Geometry: final body of the model. Coordinates: model frame, mm. Face numbers are marked on the shaded views. A direction names the side the tool comes from. Give positions to 0.01 mm unless a question says otherwise; leave off trailing zeros. Write each loop counter-clockwise with the first axis right and the second up, starting at its lowest first coordinate (ties: lowest second). Pieces come first, ordered by that corner, then holes. Notation, with made-up numbers: (-17.5, 43) -> (11.5, 43) arc R22 cw to (11.5, 80) -> close; hole circle Ø7 at (46.25, -37.75). An arc over 180 degrees is marked (long way). Answer in a Markdown table with one row per item. Add a question column.
from build123d import *

# Parameters (mm, degrees)
BOSS_EXTRUDE1_DEPTH = 60
SKETCH6_W           = 76.2
SKETCH6_H           = 139.7
BOSS_EXTRUDE3_DEPTH = 3
SKETCH7_W           = 254.695348458
SKETCH7_H           = 135.329086622
CUT_EXTRUDE1_DEPTH  = 76.2
SKETCH8_W           = 10
SKETCH8_H           = 5
CUT_EXTRUDE2_DEPTH  = 95.039099262
SKETCH9_W           = 55
SKETCH9_H           = 40
CUT_EXTRUDE3_DEPTH  = 204.2
SKETCH10_W          = 200.764393162
SKETCH10_H          = 14.388440844
CUT_EXTRUDE4_DEPTH  = 15
BOSS_EXTRUDE4_DEPTH = 4
BOSS_EXTRUDE5_DEPTH = 4


with BuildPart() as part:
    # Sketch1 → Boss-Extrude1 (new body)
    with BuildSketch(Plane.XY):
        with BuildLine():
            Line((-101.6, 101.6), (-101.6, -38.1))
            ThreePointArc((-101.6, -38.1), (-83.001280605, -83.001280605), (-38.1, -101.6))
            Line((-38.1, -101.6), (38.1, -101.6))
            ThreePointArc((38.1, -101.6), (83.001280605, -83.001280605), (101.6, -38.1))
            Line((101.6, -38.1), (101.6, 101.6))
            Line((101.6, 101.6), (-101.6, 101.6))
        make_face()
        with BuildLine():
            Line((-98.6, 98.6), (-98.6, -38.1))
            ThreePointArc((-98.6, -38.1), (-80.879960262, -80.879960262), (-38.1, -98.6))
            Line((-38.1, -98.6), (38.1, -98.6))
            ThreePointArc((38.1, -98.6), (80.879960262, -80.879960262), (98.6, -38.1))
            Line((98.6, -38.1), (98.6, 98.6))
            Line((98.6, 98.6), (-98.6, 98.6))
        make_face(mode=Mode.SUBTRACT)
    extrude(amount=BOSS_EXTRUDE1_DEPTH)

    # Sweep2: sweep along a path in Sketch5
    with BuildLine(Plane.XY.offset(60)) as sweep2_path:
        Line((-100.1, 101.6), (-100.1, -38.1))
        ThreePointArc((-100.1, -38.1), (-81.940620434, -81.940620434), (-38.1, -100.1))
        Line((-38.1, -100.1), (38.1, -100.1))
        ThreePointArc((38.1, -100.1), (81.940620434, -81.940620434), (100.1, -38.1))
        Line((100.1, -38.1), (100.1, 101.6))
    # Sketch3 → Sweep2 (sweep)
    with BuildSketch(Plane(origin=(0, 101.6, 0), x_dir=(1, 0, 0), z_dir=(0, 1, 0))):
        with BuildLine():
            Line((-38.1, -91.039099262), (-88.9, -91.039099262))
            ThreePointArc((-88.9, -91.039099262), (-95.981959893, -87.480761361), (-98.6, -80))
            Line((-98.6, -80), (-98.6, -60))
            Line((-98.6, -60), (-101.6, -60))
            Line((-101.6, -60), (-101.6, -80))
            ThreePointArc((-101.6, -80), (-98.157592659, -89.649805752), (-88.9, -94.039099262))
            Line((-88.9, -94.039099262), (-38.1, -94.039099262))
            Line((-38.1, -94.039099262), (-38.1, -91.039099262))
        make_face()
    sweep(path=sweep2_path.line)

    # Sketch6 → Boss-Extrude3 (add)
    with BuildSketch(Plane.XY.offset(94.039099262)):
        with Locations((0, 31.75)):
            Rectangle(SKETCH6_W, SKETCH6_H)
    extrude(amount=-BOSS_EXTRUDE3_DEPTH)

    # Sketch7 → Cut-Extrude1 (cut)
    with BuildSketch(Plane(origin=(0, 101.6, 0), x_dir=(1, 0, 0), z_dir=(0, 1, 0))):
        with Locations((-4.889183354, -23.374555951)):
            Rectangle(SKETCH7_W, SKETCH7_H)
    extrude(amount=-CUT_EXTRUDE1_DEPTH, mode=Mode.SUBTRACT)

    # Sketch8 → Cut-Extrude2 (cut, through all)
    with BuildSketch(Plane.XY.offset(94.039099262)):
        with Locations((0, 39.440517612)):
            Rectangle(SKETCH8_W, SKETCH8_H)
    extrude(amount=-CUT_EXTRUDE2_DEPTH, mode=Mode.SUBTRACT)

    # Sketch9 → Cut-Extrude3 (cut, through all)
    with BuildSketch(Plane(origin=(0, -101.6, 0), x_dir=(-1, 0, 0), z_dir=(0, -1, 0))):
        with Locations((0, -20)):
            Rectangle(SKETCH9_W, SKETCH9_H)
    extrude(amount=-CUT_EXTRUDE3_DEPTH, mode=Mode.SUBTRACT)

    # Sketch10 → Cut-Extrude4 (cut)
    with BuildSketch(Plane(origin=(0, 101.6, 0), x_dir=(1, 0, 0), z_dir=(0, 1, 0))):
        with Locations((0, -94.039099262)):
            Rectangle(SKETCH10_W, SKETCH10_H)
    extrude(amount=-CUT_EXTRUDE4_DEPTH, mode=Mode.SUBTRACT)

    # Sketch11 → Boss-Extrude4 (add)
    with BuildSketch(Plane(origin=(0, -98.6, 0), x_dir=(1, 0, 0), z_dir=(0, 1, 0))):
        Polygon((0, -80), (1.5, -80), (1.5, -40), (0, -40), (-1.5, -40), (-1.5, -80), align=None)
    extrude(amount=BOSS_EXTRUDE4_DEPTH)

    # Sketch12 → Boss-Extrude5 (add)
    with BuildSketch(Plane(origin=(0, 0, 91.039099262), x_dir=(-1, 0, 0), z_dir=(0, 0, -1))):
        Polygon((-1.5, -88.9), (0, -88.9), (1.5, -88.9), (1.5, 36.940517612), (-1.5, 36.940517612), align=None)
    extrude(amount=BOSS_EXTRUDE5_DEPTH)


solid = part.part
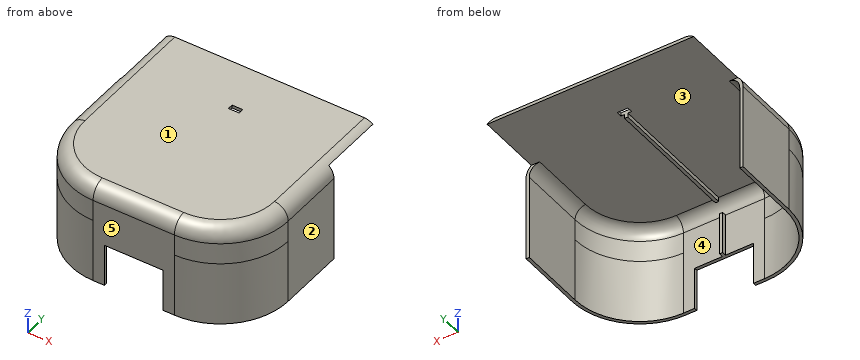
Q1. Section A-A on z = 26. Return loops of the section in (x, y), and give its area (3 significant figures).
Q2. Contact query for flat-ended pins moving along their axis: pin 1 Ø3.5 at (x, y) = (0.5, -34.5) entering from -Z; pin 2 Ø6 at (x, y) = (-77, 44) entering from -Z; pin 3 Ø23 at (x, z) = (-7.5, 45.5) entering from -Y. Output: stop coordinate, or through.
Q3. Section D-D on z = 45. Return loops of the section in (x, y), and give its area (3 significant figures).
Q4. Section C-C on x = 8. Return loops of the section in (y, z).
Q5. Access query for the marked faces 4 and 5. Directions: +Z, -Z, +X, -X, +Y, -Y. A direction counts if a zero-diameter tool reaches every point of the face in a straight line with its end or side. Return the directions, or none.
Q6. Line query: probe 1 along Y at (x, z) = (-32.5, 33); probe 2 along Z at (x, y) = (7, 8.5); probe 3 along X at (y, z) = (-66.5, 33). Output: solid intervals per line, ascending. Write a range as from..to.
Q7. Pull-direction query (Z, two-part tool) for the marked faces 1, 2 and 3; classes: +Z half, -Z half, draft (parallel to the pull), parting line (faces both ways), or undercut.
Q8. Section B-B on y = 13. Return loops of the section in (x, z), and give its area (3 significant figures).
Checks:
| question | item | result |
|---|---|---|
| 1 | outline | (-101.6, -38.1) arc R63.5 ccw to (-38.1, -101.6) -> (-27.5, -101.6) -> (-27.5, -98.6) -> (-38.1, -98.6) arc R60.5 cw to (-98.6, -38.1) -> (-98.6, 25.4) -> (-101.6, 25.4) -> close; (27.5, -101.6) -> (38.1, -101.6) arc R63.5 ccw to (101.6, -38.1) -> (101.6, 25.4) -> (98.6, 25.4) -> (98.6, -38.1) arc R60.5 cw to (38.1, -98.6) -> (27.5, -98.6) -> close |
| 1 | area | 1,030 mm^2 |
| 2 | pin 1 | z = 87.04 |
| 2 | pin 2 | z = 91.04 |
| 2 | pin 3 | y = -101.6 |
| 3 | outline | (-101.6, -38.1) arc R63.5 ccw to (-38.1, -101.6) -> (38.1, -101.6) arc R63.5 ccw to (101.6, -38.1) -> (101.6, 25.4) -> (98.6, 25.4) -> (98.6, -38.1) arc R60.5 cw to (38.1, -98.6) -> (1.5, -98.6) -> (1.5, -94.6) -> (-1.5, -94.6) -> (-1.5, -98.6) -> (-38.1, -98.6) arc R60.5 cw to (-98.6, -38.1) -> (-98.6, 25.4) -> (-101.6, 25.4) -> close |
| 3 | area | 1,210 mm^2 |
| 4 | outline | (-101.6, 40) -> (-98.6, 40) -> (-98.6, 80) arc R10.57 cw to (-88.9, 91.04) -> (86.6, 91.04) -> (86.6, 94.04) -> (-88.9, 94.04) arc R13.39 ccw to (-101.6, 80) -> close |
| 5 | face 4 | -Z, +Y |
| 5 | face 5 | +Z, -Z, +X, -X, -Y |
| 6 | probe 1 | -101.6..-98.6 |
| 6 | probe 2 | 91.04..94.04 |
| 6 | probe 3 | -94.9..-91.52, 91.52..94.9 |
| 7 | face 1 | +Z half |
| 7 | face 2 | draft |
| 7 | face 3 | -Z half |
| 8 | outline | (-101.6, 0) -> (-98.6, 0) -> (-98.6, 80) arc R10.57 cw to (-88.9, 91.04) -> (-1.5, 91.04) -> (-1.5, 87.04) -> (1.5, 87.04) -> (1.5, 91.04) -> (88.9, 91.04) arc R10.57 cw to (98.6, 80) -> (98.6, 0) -> (101.6, 0) -> (101.6, 80) arc R13.39 ccw to (88.9, 94.04) -> (-88.9, 94.04) arc R13.39 ccw to (-101.6, 80) -> close |
| 8 | area | 1,140 mm^2 |
